Build history of the part. All positions in model axes, mm. A direction names the side the tool comes from. Give positions to 0.01 mm unless a question says otherwise; leave off trailing zeros. Use a Markdown table: item, result. Add a question column.
(1) Which spindle directions (+Z, -Z, +X, -X, +Y, -Y) get a long thin tool onto all of the face, cutting with end or side? Do faces 1 (the face through (-17, 5, -1)), 2 (the face through (-0.5, 5, -17)), 3 (the face through (-4.918, 15.678, -15.617)), 4 (the face through (2.236, 7.056, 9.479)). Say none if no direction does.
(2) Wall check: line 1 (X direction, y = 5.5, z = 0); line 2 (X direction, y = 10.5, z = 12); line 3 (X direction, y = 6.25, z = 14). Give the ranges that are in metal, low to high.
(3) Flat gauge pins, fed straight in: pin 1 (6 mm diameter, centred on y = 8, z = -13.5, fed in from +X); pin 2 (4 mm diameter, centred on x = -2.5, z = -9, fed in from -Y); pin 3 (5 mm diameter, centred on x = 10, y = 8.5, fed in from +Z); pin 4 (3 mm diameter, centred on x = -12, z = -5.5, fed in from +Y). Where does each tip first touch, or does it go through?
(4) Slice it at A-A (z = -10). Count the separate pieces of the cut face and the enclosed holes in it, then the cut area to 3 significant figures.
(5) Mould opens along X. For faces 5 (the face through (-17.2, 10, 1.5)), 6 (the face through (-0.993, 4.93, -17.1)), 7 (the face through (1.553, 6.939, 9.772)) say: +X half, -X half, draft (parallel to the pull), parting line (faces both ways), or undercut.
from build123d import *

# Parameters (mm, degrees)
SKETCH2_W           = 2.532291702
SKETCH2_H           = 1
BOSS_EXTRUDE1_DEPTH = 10
FILLET1_R           = 1
BOSS_EXTRUDE2_START = 2
SKETCH3_R           = 5.25
SKETCH3_R_2         = 4.4
BOSS_EXTRUDE2_DEPTH = 9
BOSS_EXTRUDE3_START = -0.893384
BOSS_EXTRUDE3_DEPTH = 13.479999236
CIRPATTERN2_COUNT   = 4


with BuildPart() as part:
    # Sketch1 → Revolve1 (revolve)
    with BuildSketch(Plane.XY, mode=Mode.PRIVATE) as revolve1_sk:
        Polygon((15.5, 11), (15.5, 0), (16.5, 0), (16.5, 10), (16.25, 21.2), (15.75, 21.2), align=None)
    revolve(revolve1_sk.sketch.rotate(Axis((0, 0, 0), (0, 1, 0)), 90), axis=Axis((0, 0, 0), (0, 1, 0)))

    # Sketch2 → Boss-Extrude1 (add)
    with BuildSketch(Plane(origin=(0, 0, 0), x_dir=(1, 0, 0), z_dir=(0, 1, 0))):
        with Locations((16.733854149, -1.5)):
            Rectangle(SKETCH2_W, SKETCH2_H)
        with Locations((16.733854149, 1.5)):
            Rectangle(SKETCH2_W, SKETCH2_H)
        with Locations((-16.733854149, 1.5)):
            Rectangle(SKETCH2_W, SKETCH2_H)
        with Locations((-16.733854149, -1.5)):
            Rectangle(SKETCH2_W, SKETCH2_H)
        Polygon((0.5, -16.492422502), (0.5, -17.75), (1.5, -16.431676725), align=None)
        Polygon((-0.5, -17.75), (-1.5, -16.431676725), (-0.5, -16.492422502), align=None)
        Polygon((0.5, 17.75), (1.5, 16.431676725), (0.5, 16.492422502), align=None)
        Polygon((-0.5, 16.492422502), (-0.5, 17.75), (-1.5, 16.431676725), align=None)
    extrude(amount=BOSS_EXTRUDE1_DEPTH)

    # Fillet1
    fillet1_edges = [part.edges().sort_by_distance(p)[0] for p in [
        (-18, 5, -2),
        (-18, 5, 2),
        (18, 5, -2),
        (18, 5, 2),
    ]]
    fillet(fillet1_edges, radius=FILLET1_R - 0.0001)  # a hair under: the kernel refuses the full size


with BuildPart() as body_2:
    # Sketch3 → Boss-Extrude2 (new body)
    with BuildSketch(Plane(origin=(0, 0, 0), x_dir=(1, 0, 0), z_dir=(0, 1, 0)).offset(BOSS_EXTRUDE2_START)):
        with Locations(Location((0, 0, 0), (0, 0, 270))):
            Circle(SKETCH3_R)
        with Locations(Location((0, 0, 0), (0, 0, 270))):
            Circle(SKETCH3_R_2, mode=Mode.SUBTRACT)
    extrude(amount=BOSS_EXTRUDE2_DEPTH)


with BuildPart() as body_3:
    # Sketch5 → Boss-Extrude3 (new body)
    with BuildSketch(Plane(origin=(15.902515524, 0, 4.4), x_dir=(0.2666666666666668, 0, -0.9637888196533974), z_dir=(0.9637888196533975, 0, 0.2666666666666668)).offset(BOSS_EXTRUDE3_START)):
        with BuildLine():
            Line((4, 11), (4.8, 11))
            ThreePointArc((4.8, 11), (4.682488051, 7), (4.8, 3))
            Line((4.8, 3), (4.4, 3))
            ThreePointArc((4.4, 3), (4.100062422, 6.995003121), (4, 11))
        make_face()
    extrude(amount=-BOSS_EXTRUDE3_DEPTH)


with BuildPart() as cirpattern2_1:
    # CirPattern2: pattern copy
    add(body_3.part.rotate(Axis((0, 0, 0), (0, 1, 0)), 1 * 360 / CIRPATTERN2_COUNT))


with BuildPart() as cirpattern2_2:
    # CirPattern2: pattern copy
    add(body_3.part.rotate(Axis((0, 0, 0), (0, 1, 0)), 2 * 360 / CIRPATTERN2_COUNT))


with BuildPart() as cirpattern2_3:
    # CirPattern2: pattern copy
    add(body_3.part.rotate(Axis((0, 0, 0), (0, 1, 0)), 3 * 360 / CIRPATTERN2_COUNT))


with BuildPart() as part_1:
    add(part.part)

    # Combine1: union body 2, body 3, CirPattern2_1, CirPattern2_2, CirPattern2_3
    add(body_2.part)
    add(body_3.part)
    add(cirpattern2_1.part)
    add(cirpattern2_2.part)
    add(cirpattern2_3.part)


solid = part_1.part
Solution:
| question | item | result |
|---|---|---|
| 1 | face 1 | -X, +Y, -Y |
| 1 | face 2 | -Z, +Y, -Y |
| 1 | face 3 | +Y |
| 1 | face 4 | none |
| 2 | line 1 | -16.5 to -15.5, -5.25 to -4.4, 4.4 to 5.25, 15.5 to 16.5 |
| 2 | line 2 | -11.31 to -9.81, 0.83 to 1.63, 9.81 to 11.31 |
| 2 | line 3 | -8.73 to -6.65, 0.42 to 0.99, 6.65 to 8.73 |
| 3 | pin 1 | x = 12.73 |
| 3 | pin 2 | y = 3 |
| 3 | pin 3 | z = 14.7 |
| 3 | pin 4 | through |
| 4 | separate pieces | 3 |
| 4 | enclosed holes | 0 |
| 4 | area | 52.4 mm2 |
| 5 | face 5 | draft |
| 5 | face 6 | -X half |
| 5 | face 7 | undercut |
